```python
from build123d import *

# Parameters (mm, degrees)
F0_R     = 4.445
F1_DEPTH = 12.7
F2_R     = 3.81


with BuildPart() as f1:
    # F0 (on Top) → F1 (new body)
    with BuildSketch(Plane.XY):
        Circle(F0_R)
    extrude(amount=F1_DEPTH)

    # F2
    f2_edges = [f1.edges().sort_by_distance(p)[0] for p in [
        (-4.445, 0, 12.7),
    ]]
    fillet(f2_edges, radius=F2_R)

    # F3 (on Front) → F4 (revolve, cut)
    with BuildSketch(Plane.XZ):
        with BuildLine():
            Line((-2.54, 0), (0, 0))
            Line((0, 0), (0, 8.636))
            Line((0, 8.636), (0, 11.176))
            ThreePointArc((0, 11.176), (-1.796051, 10.432051), (-2.54, 8.636))
            Line((-2.54, 8.636), (-2.54, 0))
        make_face()
    revolve(axis=Axis((0, 0, 4.318), (0, 0, -1)), mode=Mode.SUBTRACT)


solid = f1.part
```
Geometry check sheet. Reference: the model listing, model coordinates, mm. Give positions to 0.01 mm unless a question says otherwise; leave off trailing zeros. Write each loop counter-clockwise with the first axis right and the second up, starting at its lowest first coordinate (ties: lowest second). Pieces come first, ordered by that corner, then holes. Notation, with made-up numbers: (47, -5.75) - (64, -5.75) arc R18 cw to (64, 14.25) - close; hole circle Ø1 at (-15, 89.25). An arc over 180 degrees is marked (long way). Use a Markdown table: item, result.
Q1. Go/stop test with flat-tipped pins: P1, Ø4, axis at x = 2.5, z = 8, coming from the -Y side; P2, Ø5, axis at x = 0, y = -2.5, coming from the +Z side. Record where each tip stops, or that it passes through.
Computed:
| item | result |
|---|---|
| P1 | stops at y = -4.42 |
| P2 | stops at z = 12.7 |
Q2. Draft check along X on faces 1 (the face through (2, -2, 0)), 2 (the face through (0.33, 2.52, 4.26)), 3 (the face through (-0.96, -4.34, 4.38)). Enter one of: pulls with the +X half, pulls with the -X half, needs draft (parallel to the pull), parting line crosses it, or undercut.
Computed:
| item | result |
|---|---|
| face 1 | needs draft |
| face 2 | undercut |
| face 3 | parting line crosses it |
Q3. Thickness scan on L1, parallel to Y at x = 0, z = 3.5 (3 decimals); L2, parallel to Y at x = 2, z = 4.5; L3, parallel to X at y = -0.75, z = 1. Record the ranges inside material, lowest first. Write a range as [from, to].
Computed:
| item | result |
|---|---|
| L1 | y = [-4.445, -2.54], [2.54, 4.445] |
| L2 | y = [-3.97, -1.57], [1.57, 3.97] |
| L3 | x = [-4.38, -2.43], [2.43, 4.38] |
Q4. Section check A-A, the plane z = 7. Enter the section's corners in (x, y) (3 decimals), then the cut area to 3 significant figures.
Computed:
| item | result |
|---|---|
| outline | circle Ø8.89 at (0, 0); hole circle Ø5.08 at (0, 0) |
| area | 41.8 mm² |
